```python
from build123d import *

# Parameters (mm, degrees)
BOSS_EXTRUDE1_DEPTH = 50
BOSS_EXTRUDE2_DEPTH = 3
BOSS_EXTRUDE3_DEPTH = 3


with BuildPart() as part:
    # Sketch6 → Boss-Extrude1 (new body)
    with BuildSketch(Plane(origin=(0, 0, 0), x_dir=(1, 0, 0), z_dir=(0, 1, 0))):
        with BuildLine():
            Line((0, 40), (-13, 40))
            Line((-13, 40), (-13, 38))
            Line((-13, 38), (-5, 38))
            Line((-5, 38), (-5, 35))
            Line((-5, 35), (-13, 35))
            Line((-13, 35), (-13, 33))
            Line((-13, 33), (-3, 33))
            Line((-3, 33), (-3, 38))
            ThreePointArc((-3, 38), (38.118237105, 0), (-3, -38))
            Line((-3, -38), (-3, -33))
            Line((-3, -33), (-13, -33))
            Line((-13, -33), (-13, -35))
            Line((-13, -35), (-5, -35))
            Line((-5, -35), (-5, -38))
            Line((-5, -38), (-13, -38))
            Line((-13, -38), (-13, -40))
            Line((-13, -40), (0, -40))
            ThreePointArc((0, -40), (40, 0), (0, 40))
        make_face()
    extrude(amount=BOSS_EXTRUDE1_DEPTH)

    # Sketch7 → Boss-Extrude2 (add)
    with BuildSketch(Plane(origin=(0, 50, 0), x_dir=(1, 0, 0), z_dir=(0, 1, 0))):
        with BuildLine():
            Line((0, -38), (-13, -38))
            Line((-13, -38), (-13, -40))
            Line((-13, -40), (0, -40))
            ThreePointArc((0, -40), (40, 0), (0, 40))
            Line((0, 40), (-13, 40))
            Line((-13, 40), (-13, 38))
            Line((-13, 38), (0, 38))
            ThreePointArc((0, 38), (38, 0), (0, -38))
        make_face()
    extrude(amount=BOSS_EXTRUDE2_DEPTH)

    # Sketch8 → Boss-Extrude3 (add)
    with BuildSketch(Plane.XZ):
        with BuildLine():
            Line((0, -40), (-13, -40))
            Line((-13, -40), (-13, -38))
            Line((-13, -38), (0, -38))
            ThreePointArc((0, -38), (38, 0), (0, 38))
            Line((0, 38), (-13, 38))
            Line((-13, 38), (-13, 40))
            Line((-13, 40), (0, 40))
            ThreePointArc((0, 40), (40, 0), (0, -40))
        make_face()
    extrude(amount=BOSS_EXTRUDE3_DEPTH)


solid = part.part
```
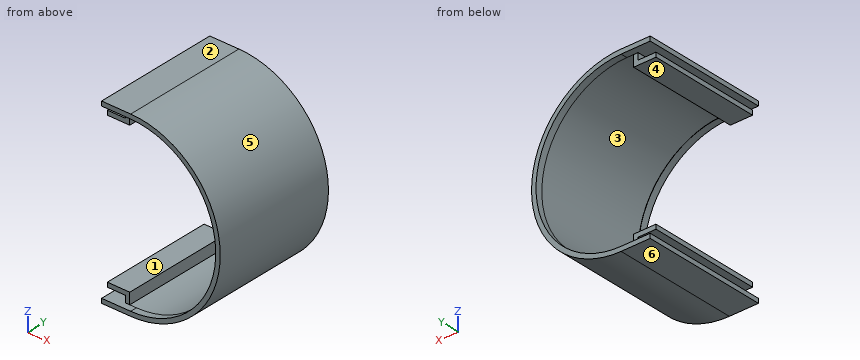
Build history of the part. All positions in model axes, mm. Face numbers are marked on the shaded views. A direction names the side the tool comes from. Give positions to 0.01 mm unless a question says otherwise; leave off trailing zeros. Loops run counter-clockwise (first coordinate to the right, second up) from the corner with the lowest first, then second, coordinate; pieces in that order, holes last. Notation, with made-up numbers: (41.25, 73) -> (71.25, 73) arc R21 ccw to (71.25, 86) -> close; hole circle Ø8 at (46, 12). An arc over 180 degrees is marked (long way). One line per question, with ' | ' between items.
Q1. Drill centre lines: line 1 along Z through (x, y) = (-3.5, 20); line 2 along Z through (x, y) = (1, 4); line 3 along X through (y, z) = (32, 20.5). Where is each one in solid material? Low to high. Write a range as [from, to].
Filled sheet:
line 1: z = [-40, -33], [33, 40] | line 2: z = [-39.99, -38.11], [38.11, 39.99] | line 3: x = [32.14, 34.35]
Q2. Pull direction Z, two halves, no side cores. Call the marked faces 4, 5 and 6: pulls with the +Z half, pulls with the -Z half, needs draft (parallel to the pull), parting line crosses it, or undercut.
Filled sheet:
face 4: undercut | face 5: parting line crosses it | face 6: pulls with the -Z half
Q3. Cut at C-C, the plane z = 0. Write the cut outline in (x, y).
Filled sheet:
outline: (38, -3) -> (40, -3) -> (40, 53) -> (38, 53) -> (38, 50) -> (38.12, 50) -> (38.12, 0) -> (38, 0) -> close
Q4. Cut at B-B, the plane x = 2. Write the cut outline in (y, z).
Filled sheet:
outline: (-3, -39.95) -> (53, -39.95) -> (53, -37.95) -> (50, -37.95) -> (50, -38.07) -> (0, -38.07) -> (0, -37.95) -> (-3, -37.95) -> close; (-3, 37.95) -> (0, 37.95) -> (0, 38.07) -> (50, 38.07) -> (50, 37.95) -> (53, 37.95) -> (53, 39.95) -> (-3, 39.95) -> close
Q5. Cut at A-A, the plane y = 13.5. Write the cut outline in (x, z).
Filled sheet:
outline: (-13, -40) -> (0, -40) arc R40 ccw to (0, 40) -> (-13, 40) -> (-13, 38) -> (-5, 38) -> (-5, 35) -> (-13, 35) -> (-13, 33) -> (-3, 33) -> (-3, 38) arc R38.12 cw (long way) to (-3, -38) -> (-3, -33) -> (-13, -33) -> (-13, -35) -> (-5, -35) -> (-5, -38) -> (-13, -38) -> close
Q6. Drop flat-ended pins along their axis: pin 1 (4 mm diameter, centred on x = -9.5, z = -35.5, fed in from +Y); pin 2 (10 mm diameter, centred on x = 26.5, y = 22, fed in from -Z); pin 3 (8 mm diameter, centred on x = 18, y = 37, fed in from +Z). Give the stop position or say it passes through.
Filled sheet:
pin 1: stops at y = 50 | pin 2: stops at z = -33.73 | pin 3: stops at z = 37.47
Q7. Cut at D-D, the plane x = 22.5. Write the cut outline in (y, z).
Filled sheet:
outline: (-3, -33.07) -> (53, -33.07) -> (53, -30.62) -> (50, -30.62) -> (50, -30.77) -> (0, -30.77) -> (0, -30.62) -> (-3, -30.62) -> close; (-3, 30.62) -> (0, 30.62) -> (0, 30.77) -> (50, 30.77) -> (50, 30.62) -> (53, 30.62) -> (53, 33.07) -> (-3, 33.07) -> close
Q8. Tool access for the marked faces 1, 2 and 3: list every direction of +Z, -Z, +X, -X, +Y, -Y with a clear straight run to the whole face (end or side of a thin tool).
Filled sheet:
face 1: -X, +Y, -Y | face 2: +Z, +X, -X, +Y, -Y | face 3: none
